Design review of the part shown in the three views and the two pictorial views. Dimensions are in mm from the part's minimum x, y and z. Coordinates: 2 decimals unless noted, no trailing zeros. Loops run counter-clockwise (first coordinate to the right, second up) from the corner with the lowest first, then second, coordinate; pieces in that order, holes last.
Q1. Add section C-C on y = 4. Give the boundary of the cut face in (x, z), and give its area (3 significant figures).
Q2. Add section D-D on x = 150. Give the boundary of the cut face in (y, z), and give its area (3 significant figures).
Q3. Add section A-A on x = 225. Give the boundary of the cut face in (y, z).
Q4. For P1, Ø6.5, axis at x = 287.5, z = 65, coming from the -Y side; P2, Ø1, axis at y = 5.5, z = 18, coming from the +X side, all flat-tipped, find the tip position at first contact; note any pin that passes through.
Q5. Wall thickness on probe 1 along Z at (x, y) = (150, 4.75); probe 2 along Z at (x, y) = (225, 5.5); probe 3 along X at (y, z) = (1.25, 70): over which ranges is each line inside the solid? List them lowest first.
Q6. Add section B-B on z = 65. Give the boundary of the cut face in (x, y), and give its area (3 significant figures).
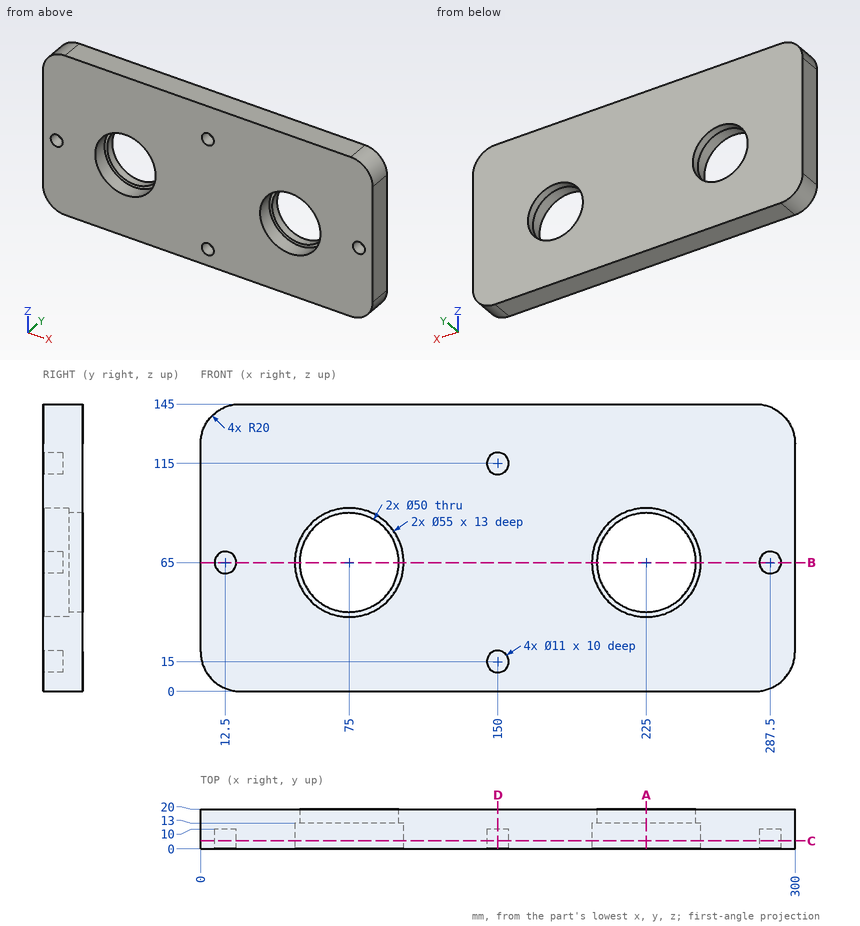
Entries:
1. outline: (0, 20) arc R20 ccw to (20, 0) - (280, 0) arc R20 ccw to (300, 20) - (300, 125) arc R20 ccw to (280, 145) - (20, 145) arc R20 ccw to (0, 125) - close; hole circle Ø11 at (12.5, 65); hole circle Ø55 at (75, 65); hole circle Ø11 at (150, 15); hole circle Ø11 at (150, 115); hole circle Ø55 at (225, 65); hole circle Ø11 at (287.5, 65)
1. area: 38,000 mm2
2. outline: (0, 0) - (20, 0) - (20, 145) - (0, 145) - (0, 120.5) - (10, 120.5) - (10, 109.5) - (0, 109.5) - (0, 20.5) - (10, 20.5) - (10, 9.5) - (0, 9.5) - close
2. area: 2,680 mm2
3. outline: (0, 0) - (20, 0) - (20, 40) - (13, 40) - (13, 37.5) - (0, 37.5) - close; (0, 92.5) - (13, 92.5) - (13, 90) - (20, 90) - (20, 145) - (0, 145) - close
4. P1: stops at y = 10
4. P2: stops at x = 299.94
5. probe 1: z = 0 to 9.5, 20.5 to 109.5, 120.5 to 145
5. probe 2: z = 0 to 37.5, 92.5 to 145
5. probe 3: x = 0 to 10.21, 14.79 to 47.96, 102.04 to 197.96, 252.04 to 285.21, 289.79 to 300
6. outline: (0, 0) - (7, 0) - (7, 10) - (18, 10) - (18, 0) - (47.5, 0) - (47.5, 13) - (50, 13) - (50, 20) - (0, 20) - close; (100, 13) - (102.5, 13) - (102.5, 0) - (197.5, 0) - (197.5, 13) - (200, 13) - (200, 20) - (100, 20) - close; (250, 13) - (252.5, 13) - (252.5, 0) - (282, 0) - (282, 10) - (293, 10) - (293, 0) - (300, 0) - (300, 20) - (250, 20) - close
6. area: 3,650 mm2
